Source: CAD feature listing. Evaluate the final solid. Frame: model axes, mm. Give positions to 0.01 mm unless a question says otherwise; leave off trailing zeros. Order: outer loops, then holes, each group sorted by start corner. A loop starts at its lowest first (then second) coordinate and runs counter-clockwise, first axis right, second up.
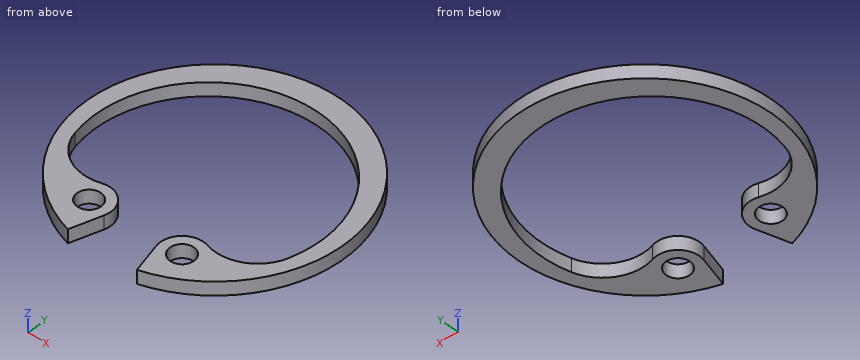
from build123d import *

# Parameters (mm, degrees)
ESQUISSE1_R        = 0.75480164
BOSS_EXTRU_1_DEPTH = 0.8521954


with BuildPart() as part:
    # Esquisse1 → Boss.-Extru.1 (new body)
    with BuildSketch(Plane.XY.offset(-0.0184023)):
        with BuildLine():
            Line((-2.218240991, -7.772182242), (-1.669933881, -5.847622743))
            ThreePointArc((-1.669933881, -5.847622743), (-2.031629427, -4.49557761), (-3.39387782, -4.174440527))
            ThreePointArc((-3.39387782, -4.174440527), (-5.528675736, -3.967277273), (-6.85337913, -2.280434165))
            ThreePointArc((-6.85337913, -2.280434165), (0, 6.648799775), (6.85337913, -2.280434165))
            ThreePointArc((6.85337913, -2.280434165), (5.528675736, -3.967277273), (3.39387782, -4.174440527))
            ThreePointArc((3.39387782, -4.174440527), (2.031629427, -4.49557761), (1.669933881, -5.847622743))
            Line((1.669933881, -5.847622743), (2.218240991, -7.772182242))
            ThreePointArc((2.218240991, -7.772182242), (0, 8.109706175), (-2.218240991, -7.772182242))
        make_face()
        with Locations((2.981265606, -5.47402426)):
            Circle(ESQUISSE1_R, mode=Mode.SUBTRACT)
        with Locations((-2.981265606, -5.47402426)):
            Circle(ESQUISSE1_R, mode=Mode.SUBTRACT)
    extrude(amount=-BOSS_EXTRU_1_DEPTH)


solid = part.part
(1) Section B-B, the plane x = 6.5. Return loops of the section in (y, z), plus the area to 3 significant figures.
(2) Section A-A, the plane y = 5.5. Return loops of the section in (x, z), plus the area to 3 significant figures.
(3) Line query: line 1 along Y through (x, z) = (3, -0.15); line 2 along Y through (x, z) = (-2.5, -0.6); line 3 along X through (y, z) = (-5, -0.8). Output: solid intervals per line, ascending.
(4) Section C-C, the plane z = -0.3. Return loops of the section in (x, y).
(5) Section D-D, the plane x = 0. Return loops of the section in (y, z).
Checks:
1. outline: (-4.81, -0.87) - (-3.07, -0.87) - (-3.07, -0.02) - (-4.81, -0.02) - close; (2.4, -0.87) - (4.84, -0.87) - (4.84, -0.02) - (2.4, -0.02) - close
1. area: 3.57 mm2
2. outline: (-5.95, -0.87) - (-3.87, -0.87) - (-3.87, -0.02) - (-5.95, -0.02) - close; (3.87, -0.87) - (5.95, -0.87) - (5.95, -0.02) - (3.87, -0.02) - close
2. area: 3.55 mm2
3. line 1: y = -7.51 to -6.23, -4.72 to -4.11, 5.98 to 7.53
3. line 2: y = -7.69 to -6.06, -4.89 to -4.2, 6.19 to 7.71
3. line 3: x = -6.36 to -3.57, -2.39 to -1.7, 1.7 to 2.39, 3.57 to 6.36
4. outline: (-6.85, -2.28) arc R7.09 cw (long way) to (6.85, -2.28) arc R2.73 cw to (3.39, -4.17) arc R1.36 ccw to (1.67, -5.85) - (2.22, -7.77) arc R8.1 ccw (long way) to (-2.22, -7.77) - (-1.67, -5.85) arc R1.36 ccw to (-3.39, -4.17) arc R2.73 cw to start; hole circle Ø1.51 at (-2.98, -5.47); hole circle Ø1.51 at (2.98, -5.47)
5. outline: (6.65, -0.87) - (8.11, -0.87) - (8.11, -0.02) - (6.65, -0.02) - close
